from build123d import *

# Parameters (mm, degrees)
F1_DEPTH = 25


with BuildPart() as f1:
    # F0 (on Front) → F1 (new body)
    with BuildSketch(Plane.XZ):
        with BuildLine():
            Line((-40, 0), (0, 0))
            Line((0, 0), (40, 0))
            Line((40, 0), (40, 10.122449))
            Line((40, 10.122449), (30, 10.122449))
            Line((30, 10.122449), (30, 47.020409))
            Line((30, 47.020409), (18.897959, 47.020409))
            ThreePointArc((18.897959, 47.020409), (0, 28.12245), (-18.897959, 47.020409))
            Line((-18.897959, 47.020409), (-30, 47.020409))
            Line((-30, 47.020409), (-30, 10.122449))
            Line((-30, 10.122449), (-40, 10.122449))
            Line((-40, 10.122449), (-40, 0))
        make_face()
    extrude(amount=F1_DEPTH)


solid = f1.part
Could you check a few things on this model? Use its own coordinates, in mm. A direction names the side the tool comes from. Round coordinates to 2 decimals unless told otherwise and drop trailing zeros. Write each loop counter-clockwise with the first axis right and the second up, starting at its lowest first coordinate (ties: lowest second). Pieces come first, ordered by that corner, then holes. Notation, with made-up numbers: (74, 3.5) - (113, 3.5) arc R31 cw to (113, 36.5) - close; hole circle Ø9 at (76.5, 89.25). An arc over 180 degrees is marked (long way). Put each result on its own line as item: value. Start each with the question number.
(1) I want a section at B-B, the plane z = 24. Please give me the cut outline in (x, y).
(2) Will these pins go through, and if not, where does the flat tip stop? pin 1 (7.5 mm diameter, centred on y = -15.5, z = 31.5, fed in from -X); pin 2 (10 mm diameter, centred on y = -19, z = 30, fed in from +X); pin 3 (8 mm diameter, centred on x = 36, y = -8.5, fed in from +Z).
(3) I want a section at A-A, the plane y = -14.75. Please give me the cut outline in (x, z).
(4) I need wall thicknesses on probe 1 along X at (y, z) = (-13.25, 18); probe 2 along Z at (x, y) = (35.5, -3); probe 3 along X at (y, z) = (-4.25, 37.5). Which ranges of each line are inside material? Lowest first, please.
(5) For faces 1 (the flat face through (40, -12, 5)), 2 (the flat face through (-30, -12, 29)), 3 (the flat face through (30, -12, 28)), which set-ups out of +Z, -Z, +X, -X, +Y, -Y let a thin tool reach every point of the face, with its end or its side?
(6) I want a section at C-C, the plane x = -32. Please give me the cut outline in (y, z), plus the area to 3 significant figures.
Here are the results:
1. outline: (-30, -25) - (30, -25) - (30, 0) - (-30, 0) - close
2. pin 1: stops at x = -30
2. pin 2: stops at x = 30
2. pin 3: stops at z = 10.12
3. outline: (-40, 0) - (40, 0) - (40, 10.12) - (30, 10.12) - (30, 47.02) - (18.9, 47.02) arc R18.9 cw to (-18.9, 47.02) - (-30, 47.02) - (-30, 10.12) - (-40, 10.12) - close
4. probe 1: x = -30 to 30
4. probe 2: z = 0 to 10.12
4. probe 3: x = -30 to -16.32, 16.32 to 30
5. face 1: +Z, -Z, +X, +Y, -Y
5. face 2: +Z, -X, +Y, -Y
5. face 3: +Z, +X, +Y, -Y
6. outline: (-25, 0) - (0, 0) - (0, 10.12) - (-25, 10.12) - close
6. area: 253 mm^2
